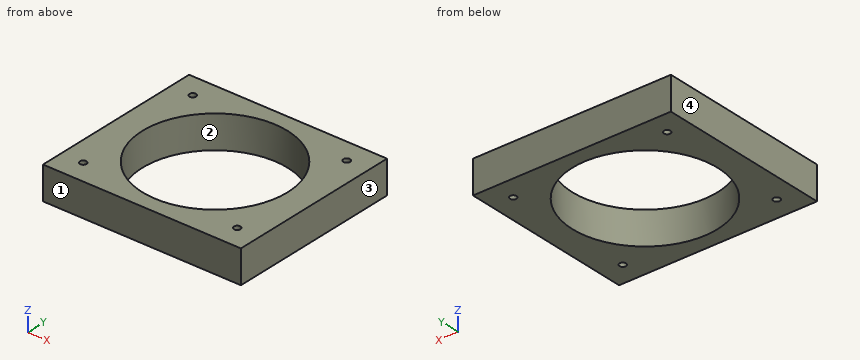
Autodesk Inventor part; units mm, degrees
ref_plane "YZ Plane" through (0, 0, 0) normal (1, 0, 0) x (0, 1, 0)
ref_plane "XZ Plane" through (0, 0, 0) normal (0, 1, 0) x (-1, 0, 0)
ref_plane "XY Plane" through (0, 0, 0) normal (0, 0, 1) x (1, 0, 0)
sketch "スケッチ1" plane through (0, 0, 0) normal (0, 0, 1) x (1, 0, 0)
  circle A0 centre (0, 0) radius 40
  line L0 (-45, 40) -> (45, 40)
  line L1 (45, 40) -> (45, -40)
  line L2 (45, -40) -> (-45, -40)
  line L3 (-45, -40) -> (-45, 40)
  line L4 (-45, 40) -> (45, -40) construction
  line L5 (45, 40) -> (-45, -40) construction
  circle A1 centre (0, 0) radius 33
  dimension "d0" = 80
  dimension "d1" = 90
  dimension "d2" = 80
  dimension "d3" = 66
extrude "押し出し1" add sketch "スケッチ1" along normal blind 15
sketch "スケッチ2" plane through (0, 0, 15) normal (0, 0, 1) x (1, 0, 0)
  line L0 (-45, 40) -> (-35, 40)
  line L1 (-35, 40) -> (-35, 30)
  line L2 (-35, 30) -> (-45, 30)
  line L3 (-45, 30) -> (-45, 40)
  line L4 (-45, -40) -> (-35, -40)
  line L5 (-35, -40) -> (-35, -30)
  line L6 (-35, -30) -> (-45, -30)
  line L7 (-45, -30) -> (-45, -40)
  line L8 (45, -40) -> (35, -40)
  line L9 (35, -40) -> (35, -30)
  line L10 (35, -30) -> (45, -30)
  line L11 (45, -30) -> (45, -40)
  line L12 (45, 40) -> (35, 40)
  line L13 (35, 40) -> (35, 30)
  line L14 (35, 30) -> (45, 30)
  line L15 (45, 30) -> (45, 40)
  dimension "d6" = 10
  dimension "d7" = 10
  dimension "d8" = 10
  dimension "d9" = 10
  dimension "d10" = 10
  dimension "d11" = 10
  dimension "d12" = 10
hole "穴1" at (-35, 30, 15) at (-35, -30, 15) at (35, -30, 15) at (35, 30, 15) direction (0, 0, -1) diameter 3 depth 15 tip angle 118
properties part number "知能ロボコン発射筒スペーサ"
Input: part model. Units: mm. Frame: model coordinates. Face numbers are marked on the shaded views. Round coordinates to 2 decimals unless told otherwise and drop trailing zeros. Order: outer loops, then holes, each group sorted by start corner. A loop starts at its lowest first (then second) coordinate and runs counter-clockwise, first axis right, second up.
1. Cut plane A-A, the plane y = 0. Output: boundary loops of the cut face in (x, z), then the cut area to 3 significant figures.
The answers:
outline: (-45, 0) - (-33, 0) - (-33, 15) - (-45, 15) - close; (33, 0) - (45, 0) - (45, 15) - (33, 15) - close
area: 360 mm2
2. Material intervals for line 1 (Y direction, x = 35, z = 5.75); line 2 (Y direction, x = 0, z = 3.5); line 3 (X direction, y = -30, z = 7.5), sorted ascending.
The answers:
line 1: y = -40 to -31.5, -28.5 to 28.5, 31.5 to 40
line 2: y = -40 to -33, 33 to 40
line 3: x = -45 to -36.5, -33.5 to -13.75, 13.75 to 33.5, 36.5 to 45
3. Cut plane B-B, the plane x = 35. Output: boundary loops of the cut face in (y, z).
The answers:
outline: (-40, 0) - (-31.5, 0) - (-31.5, 15) - (-40, 15) - close; (-28.5, 0) - (28.5, 0) - (28.5, 15) - (-28.5, 15) - close; (31.5, 0) - (40, 0) - (40, 15) - (31.5, 15) - close
4. Cut plane C-C, the plane z = 7.5. Output: boundary loops of the cut face in (x, y), then the cut area to 3 significant figures.
The answers:
outline: (-45, -40) - (45, -40) - (45, 40) - (-45, 40) - close; hole circle Ø3 at (-35, -30); hole circle Ø3 at (-35, 30); hole circle Ø66 at (0, 0); hole circle Ø3 at (35, -30); hole circle Ø3 at (35, 30)
area: 3,750 mm2
5. Mould query, pull axis X, two halves, no side actions, for the marked faces 1, 2, 3 and 4. Classes: released by +X, released by -X, zero draft, split by the parting line, or undercut.
The answers:
face 1: zero draft
face 2: undercut
face 3: released by +X
face 4: released by -X
6. Cut plane D-D, the plane x = 0. Output: boundary loops of the cut face in (y, z).
The answers:
outline: (-40, 0) - (-33, 0) - (-33, 15) - (-40, 15) - close; (33, 0) - (40, 0) - (40, 15) - (33, 15) - close
